Part model, mm, in its own coordinate system. Face numbers are marked on the shaded views. A direction names the side the tool comes from. Give positions to 0.01 mm unless a question says otherwise; leave off trailing zeros. Loops run counter-clockwise (first coordinate to the right, second up) from the corner with the lowest first, then second, coordinate; pieces in that order, holes last. Notation, with made-up numbers: (10.5, 44) -> (67.5, 44) arc R38 ccw to (67.5, 83) -> close; hole circle Ø1 at (-17.5, 24.5). An arc over 180 degrees is marked (long way). One line per question, with ' | ' between items.
```python
from build123d import *

# Parameters (mm, degrees)
F0_W     = 55
F0_H     = 35
F1_DEPTH = 40
F2_W     = 30
F2_H     = 17.0720907301
F3_DEPTH = 20
F4_R     = 5
F5_DEPTH = 40.001


# Not quite as in the source:
# - a feature names something its author has since deleted; it is built from what else it names


with BuildPart() as f1:
    # F0 (on Front) → F1 (new body)
    with BuildSketch(Plane.XZ):
        with Locations((27.5, -17.5)):
            Rectangle(F0_W, F0_H)
    extrude(amount=F1_DEPTH)

    # F2 (on face) → F3 (cut)
    with BuildSketch(Plane.XZ.offset(40)):
        with Locations((40, -26.463954635)):
            Rectangle(F2_W, F2_H)
    extrude(amount=-F3_DEPTH, mode=Mode.SUBTRACT)

    # F4 (on Front) → F5 (cut, through all)
    with BuildSketch(Plane.XZ):
        with Locations((40, -27)):
            Circle(F4_R)
    extrude(amount=F5_DEPTH, mode=Mode.SUBTRACT)


solid = f1.part
```
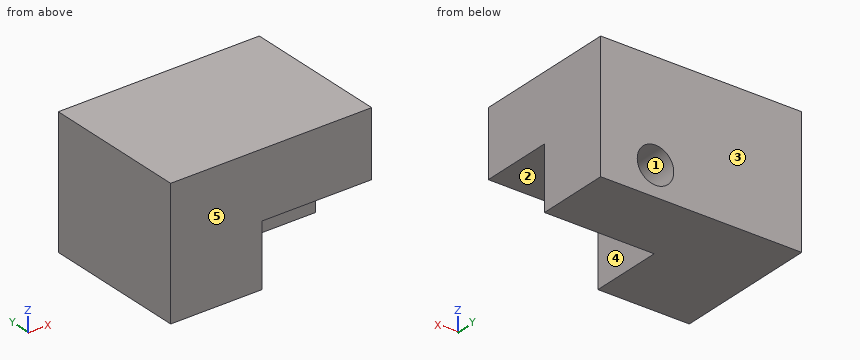
1) Pin check, flat tips, straight feed: P1, Ø13.5, axis at y = -31.5, z = -24, coming from the +X side; P2, Ø8.5, axis at x = 38, z = -28.5, coming from the -Y side; P3, Ø6, axis at x = 36, y = -29.5, coming from the -Z side. Stop position of each tip, or through.
Found:
P1: x = 55 | P2: y = -20 | P3: z = -17.93
2) Saw through at C-C (y = -14). Give the cut face in (x, z).
Found:
outline: (0, -35) -> (55, -35) -> (55, 0) -> (0, 0) -> close; hole circle Ø10 at (40, -27)
3) Drill centre lines: line 1 (Z direction, x = 40, y = -8); line 2 (X direction, y = -4, z = -27); line 3 (Z direction, x = 41.5, y = -33.5). Where is each one in solid material? Low to high.
Found:
line 1: -35 to -32, -22 to 0 | line 2: 0 to 35, 45 to 55 | line 3: -17.93 to 0
4) Tool access for the marked faces 4 and 5: list every direction of +Z, -Z, +X, -X, +Y, -Y with a clear straight run to the whole face (end or side of a thin tool).
Found:
face 4: -Z, +X, -Y | face 5: +Z, -Z, +X, -X, -Y
5) Pull direction Z, two halves, no side cores. Call the marked faces 1, 2 and 3: pulls with the +Z half, pulls with the -Z half, needs draft (parallel to the pull), parting line crosses it, or undercut.
Found:
face 1: undercut | face 2: pulls with the -Z half | face 3: needs draft
6) Saw through at A-A (x = 40). Give the cut face in (y, z).
Found:
outline: (-40, -17.93) -> (-20, -17.93) -> (-20, -22) -> (0, -22) -> (0, 0) -> (-40, 0) -> close; (-20, -35) -> (0, -35) -> (0, -32) -> (-20, -32) -> close
7) Saw through at D-D (y = -22.5). Give the cut face in (x, z), and give its area (3 significant figures).
Found:
outline: (0, -35) -> (25, -35) -> (25, -17.93) -> (55, -17.93) -> (55, 0) -> (0, 0) -> close | area: 1,410 mm2
8) Saw through at B-B (z = -27). Give the cut face in (x, y), and give its area (3 significant figures).
Found:
outline: (0, -40) -> (25, -40) -> (25, -20) -> (35, -20) -> (35, 0) -> (0, 0) -> close; (45, -20) -> (55, -20) -> (55, 0) -> (45, 0) -> close | area: 1,400 mm2
